Design review of the part shown in the three views and the two pictorial views. Dimensions are in mm from the part's minimum x, y and z. A direction names the side the tool comes from. Round coordinates to 2 decimals unless told otherwise and drop trailing zeros. Loops run counter-clockwise (first coordinate to the right, second up) from the corner with the lowest first, then second, coordinate; pieces in that order, holes last. Notation, with made-up numbers: (-22.75, 26) -> (-13.75, 26) arc R26 cw to (-13.75, 43) -> close; hole circle Ø10 at (76, 65). An arc over 180 degrees is marked (long way). Return JSON: item names as keys, results as strings. Group by question number.
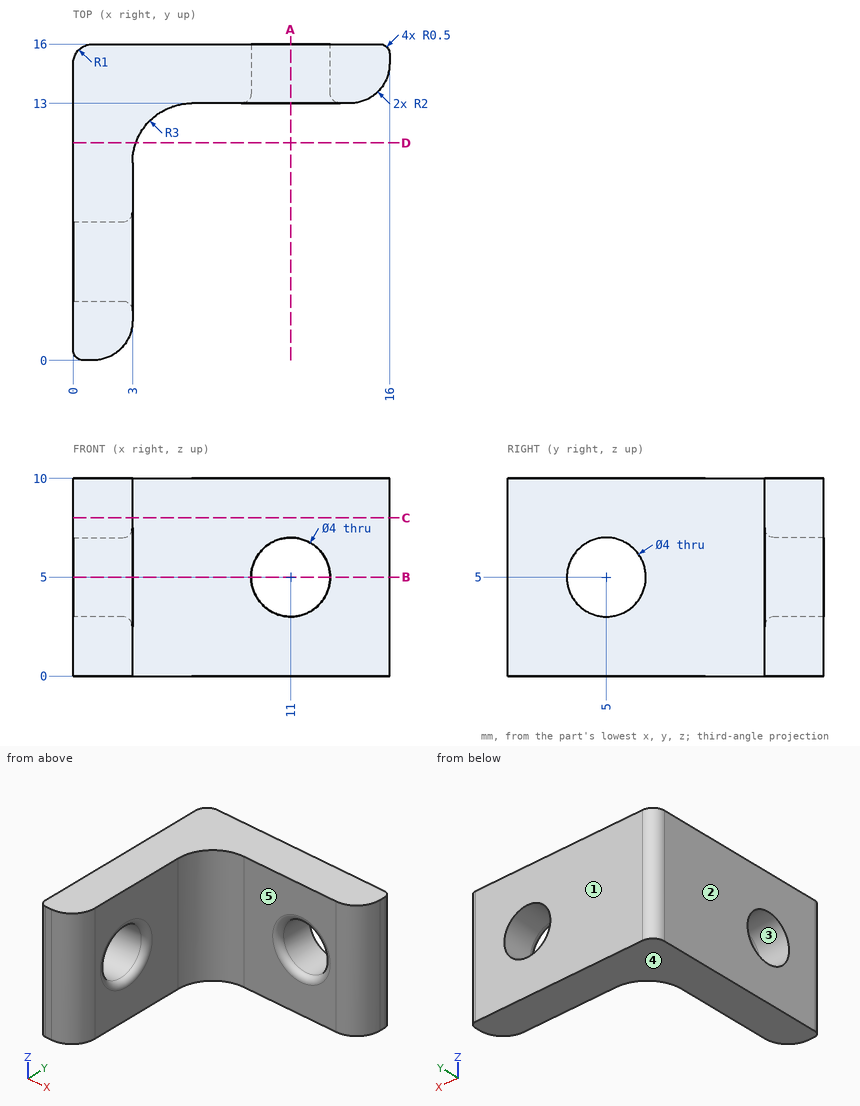
1. We need section D-D, the plane y = 11. Write out the cut boundary in (x, z).
2. For P1, Ø1, axis at x = 14, z = 8.5, coming from the -Y side; P2, Ø2.5, axis at y = 7, z = 7, coming from the +X side; P3, Ø6, axis at x = 5, z = 1.5, coming from the -Y side, all flat-tipped, find the tip position at first contact; note any pin that passes through.
3. We need section B-B, the plane z = 5. Write out the cut boundary in (x, y), then the cut area to 3 significant figures.
4. Tool access review of the marked faces 4 and 5: name each direction out of +Z, -Z, +X, -X, +Y, -Y from which nothing blocks a thin tool from reaching the whole face with its end or side.
5. We need section C-C, the plane z = 8. Write out the cut boundary in (x, y).
6. Draft analysis for pull direction Y (two halves, no side actions). For the marked faces 1, 2 and 3, state which applies: pulls with the +Y half, pulls with the -Y half, needs draft (parallel to the pull), parting line crosses it, or undercut.
7. We need section A-A, the plane x = 11. Write out the cut boundary in (y, z).
8. Wall thickness on line 1 (Z direction, x = 11, y = 14.45); line 2 (X direction, y = 14.85, z = 5); line 3 (Y direction, x = 6.5, z = 6.5): over which ranges is each line inside the solid? List them lowest first.
Check sheet entries:
{
 "1": {"outline": "(0, 0) -> (3.17, 0) -> (3.17, 10) -> (0, 10) -> close"},
 "2": {"P1": "stops at y = 13", "P2": "stops at x = 3", "P3": "stops at y = 0.27"},
 "3": {"outline": "(0, 0.5) arc R0.5 ccw to (0.5, 0) -> (1, 0) arc R2 ccw to (3, 2) -> (3, 2.5) arc R0.5 ccw to (2.5, 3) -> (0, 3) -> close; (0, 7) -> (2.5, 7) arc R0.5 ccw to (3, 7.5) -> (3, 10) arc R3 cw to (6, 13) -> (8.5, 13) arc R0.5 ccw to (9, 13.5) -> (9, 16) -> (1, 16) arc R1 ccw to (0, 15) -> close; (13, 13.5) arc R0.5 ccw to (13.5, 13) -> (14, 13) arc R2 ccw to (16, 15) -> (16, 15.5) arc R0.5 ccw to (15.5, 16) -> (13, 16) -> close", "area": "62.7 mm²"},
 "4": {"face 4": "-Z, +X, -X, +Y, -Y", "face 5": "+Z, -Z, +X, -Y"},
 "5": {"outline": "(0, 0.5) arc R0.5 ccw to (0.5, 0) -> (1, 0) arc R2 ccw to (3, 2) -> (3, 10) arc R3 cw to (6, 13) -> (14, 13) arc R2 ccw to (16, 15) -> (16, 15.5) arc R0.5 ccw to (15.5, 16) -> (1, 16) arc R1 ccw to (0, 15) -> close"},
 "6": {"face 1": "pulls with the +Y half", "face 2": "needs draft", "face 3": "undercut"},
 "7": {"outline": "(13, 0) -> (16, 0) -> (16, 3) -> (13.5, 3) arc R0.5 ccw to (13, 2.5) -> close; (13, 7.5) arc R0.5 ccw to (13.5, 7) -> (16, 7) -> (16, 10) -> (13, 10) -> close"},
 "8": {"line 1": "z = 0 to 3, 7 to 10", "line 2": "x = 0 to 9, 13 to 15.99", "line 3": "y = 13 to 16"}
}
